from build123d import *

# Parameters (mm, degrees)
BOSS_EXTRUDE1_DEPTH = 6.35


with BuildPart() as part:
    # Sketch1 → Boss-Extrude1 (new body)
    with BuildSketch(Plane(origin=(0, 0, 0), x_dir=(1, 0, 0), z_dir=(0, 1, 0))):
        with BuildLine():
            Line((53.34, 3.137679315), (53.34, 9.487679315))
            Line((53.34, 9.487679315), (59.69, 9.487679315))
            Line((59.69, 9.487679315), (59.69, 3.137679315))
            Line((59.69, 3.137679315), (60.706, 3.137679315))
            Line((60.706, 3.137679315), (60.706, 0))
            Line((60.706, 0), (60.706, -6.35))
            Line((60.706, -6.35), (55.225149786, -6.35))
            ThreePointArc((55.225149786, -6.35), (31.627279146, -30.348844293), (0, -18.837144157))
            Line((0, -18.837144157), (0, 0))
            ThreePointArc((0, 0), (24.765, -24.765), (49.53, 0))
            Line((49.53, 0), (49.53, 3.137679315))
            Line((49.53, 3.137679315), (53.34, 3.137679315))
        make_face()
    extrude(amount=BOSS_EXTRUDE1_DEPTH)


solid = part.part
Can you work these out from the model? Positions are in its coordinate system, mm. A direction names the side the tool comes from. Give positions to 0.01 mm unless a question says otherwise; leave off trailing zeros. Loops run counter-clockwise (first coordinate to the right, second up) from the corner with the lowest first, then second, coordinate; pieces in that order, holes last. Notation, with made-up numbers: (10.5, 38.5) -> (56.5, 38.5) arc R18 ccw to (56.5, 62.5) -> close; hole circle Ø11 at (-29.75, 14). An arc over 180 degrees is marked (long way). Use one line per item in the form item = value.
1) We'd pull the mould along X, two halves only. Please class faces 1 (the face through (59.69, 3, -6)), 2 (the face through (24.22, 3.13, 24.76)), 3 (the face through (51, 3, -3.138)): released by +X, released by -X, zero draft, split by the parting line, or undercut.
Answers:
face_1 = released by +X
face_2 = undercut
face_3 = zero draft
2) Will these pins go through, and if not, where does the flat tip stop? pin 1 (3 mm diameter, centred on y = 5, z = 25, fed in from +X); pin 2 (3 mm diameter, centred on y = 5.5, z = 15, fed in from +X); pin 3 (1.9 mm diameter, centred on y = 2, z = -5.5, fed in from +X).
Answers:
pin_1 = 45.16
pin_2 = 52.8
pin_3 = 59.69
3) If we section it at A-A (z = 9): Please give me the cut outline in (x, y), plus the area to 3 significant figures.
Answers:
outline = (0, 0) -> (1.69, 0) -> (1.69, 6.35) -> (0, 6.35) -> close; (47.84, 0) -> (54.55, 0) -> (54.55, 6.35) -> (47.84, 6.35) -> close
area = 53.4 mm²
4) For faces 4 (the face through (60.706, 3, 2)), 5 (the face through (58, 3, 6.35)), 6 (the face through (53.34, 3, -6)), which set-ups out of +Z, -Z, +X, -X, +Y, -Y let a thin tool reach every point of the face, with its end or its side?
Answers:
face_4 = +Z, -Z, +X, +Y, -Y
face_5 = +Z, +X, +Y, -Y
face_6 = -Z, -X, +Y, -Y
5) If we section it at B-B (y = 4.5): Please give me the cut outline in (x, z) (3 decimals).
Answers:
outline = (0, 0) arc R24.765 cw to (49.53, 0) -> (49.53, -3.138) -> (53.34, -3.138) -> (53.34, -9.488) -> (59.69, -9.488) -> (59.69, -3.138) -> (60.706, -3.138) -> (60.706, 6.35) -> (55.225, 6.35) arc R31.115 ccw to (0, 18.837) -> close
6) I need wall thicknesses on line 1 along X through (y, z) = (0.75, -3); line 2 along X through (y, z) = (5, 18); line 3 along X through (y, z) = (4.5, 5). Which ranges of each line are inside material? Lowest first, please.
Answers:
line_1 = 49.53 to 60.71
line_2 = 0 to 7.76, 41.77 to 50.14
line_3 = 0 to 0.51, 49.02 to 60.71
7) If we section it at C-C (z = 2): Please give me the cut outline in (x, y).
Answers:
outline = (0, 0) -> (0.08, 0) -> (0.08, 6.35) -> (0, 6.35) -> close; (49.45, 0) -> (60.71, 0) -> (60.71, 6.35) -> (49.45, 6.35) -> close
8) If we section it at D-D (x = 35.5): Please give me the cut outline in (y, z), plus the area to 3 significant figures.
Answers:
outline = (0, 22.32) -> (6.35, 22.32) -> (6.35, 29.2) -> (0, 29.2) -> close
area = 43.7 mm²
